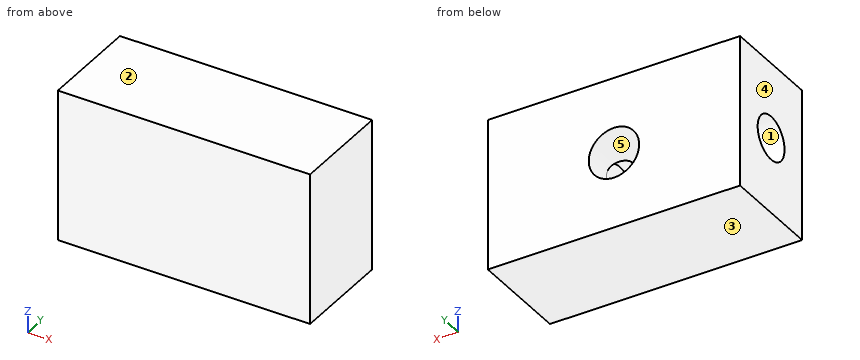
```python
from build123d import *

# Parameters (mm, degrees)
F0_W     = 127
F0_H     = 76.2
F1_DEPTH = 50.8
F2_R     = 12.7
F3_DEPTH = 38.1
F4_R     = 10.982907
F5_DEPTH = 76.2


with BuildPart() as f1:
    # F0 (on Front) → F1 (new body)
    with BuildSketch(Plane.XZ):
        with Locations((3.876453, -23.385659)):
            Rectangle(F0_W, F0_H)
    extrude(amount=F1_DEPTH)

    # F2 (on face) → F3 (cut)
    with BuildSketch(Plane(origin=(0, 0, 0), x_dir=(-1, 0, 0), z_dir=(0, 1, 0))):
        with Locations((-3.876453, -23.385659)):
            Circle(F2_R)
    extrude(amount=-F3_DEPTH, mode=Mode.SUBTRACT)

    # F4 (on face) → F5 (cut)
    with BuildSketch(Plane(origin=(-59.623547, 0, 0), x_dir=(0, -1, 0), z_dir=(-1, 0, 0))):
        with Locations((25.4, -23.385659)):
            Circle(F4_R)
    extrude(amount=-F5_DEPTH, mode=Mode.SUBTRACT)


solid = f1.part
```
Geometry check sheet. Reference: the model listing, model coordinates, mm. Face numbers are marked on the shaded views. A direction names the side the tool comes from. Coordinates: 2 decimals unless noted, no trailing zeros. Write each loop counter-clockwise with the first axis right and the second up, starting at its lowest first coordinate (ties: lowest second). Pieces come first, ordered by that corner, then holes. Notation, with made-up numbers: (77.5, 77) -> (108.5, 77) arc R11 ccw to (108.5, 97) -> close; hole circle Ø7 at (25, 12). An arc over 180 degrees is marked (long way). Use CSV: the item, a comma, the result in double quotes. Start each with the question number.
Item 1: Cross-section at B-B, the plane y = -10.5. Record the cut outline in (x, z), plus the area to 3 significant figures.
Item 2: Thickness scan on line 1 (X direction, y = -12, z = -23); line 2 (Z direction, x = -25.5, y = -25.4); line 3 (X direction, y = -9, z = -25.5). Record the ranges inside material, lowest first.
Item 3: Mould release check, pull along Z, two halves, no side actions. Record for the marked faces 3, 4 and 5: released by +Z, released by -Z, zero draft, split by the parting line, or undercut.
Item 4: Cross-section at A-A, the plane z = -19. Record the cut outline in (x, y).
Item 5: Depth check by flat-ended pin: pin 1 Ø6.5 at (y, z) = (-28.5, -18) entering from -X; pin 2 Ø7.5 at (x, z) = (2.5, -29) entering from +Y. Enter the tip coordinate at first touch or a pass-through.
Item 6: Cross-section at C-C, the plane x = -27. Record the cut outline in (y, z), plus the area to 3 significant figures.
Item 7: Cross-section at D-D, the plane y = -25.4. Record the cut outline in (x, z), plus the area to 3 significant figures.
Item 8: Set-up check for the marked faces 1 and 2: record each of +Z, -Z, +X, -X, +Y, -Y from which the full face is reachable in a straight line by a thin tool's end or side.
Answers:
1,outline,"(-59.62, -61.49) -> (67.38, -61.49) -> (67.38, 14.71) -> (-59.62, 14.71) -> close; hole circle Ø25.4 at (3.88, -23.39)"
1,area,"9,170 mm^2"
2,line 1,"-59.62 to -8.82, 16.57 to 67.38"
2,line 2,"-61.49 to -34.37, -12.4 to 14.71"
2,line 3,"-59.62 to -8.65, 16.4 to 67.38"
3,face 3,"released by -Z"
3,face 4,"zero draft"
3,face 5,"undercut"
4,outline,"(-59.62, -50.8) -> (67.38, -50.8) -> (67.38, 0) -> (15.8, 0) -> (15.8, -15.33) -> (16.58, -15.33) -> (16.58, -35.47) -> (15.8, -35.47) -> (15.8, -38.1) -> (-8.04, -38.1) -> (-8.04, -35.47) -> (-59.62, -35.47) -> close; (-59.62, -15.33) -> (-8.04, -15.33) -> (-8.04, 0) -> (-59.62, 0) -> close"
5,pin 1,"x = 16.58"
5,pin 2,"y = -38.1"
6,outline,"(-50.8, -61.49) -> (0, -61.49) -> (0, 14.71) -> (-50.8, 14.71) -> close; hole circle Ø21.97 at (-25.4, -23.39)"
6,area,"3,490 mm^2"
7,outline,"(-59.62, -61.49) -> (67.38, -61.49) -> (67.38, 14.71) -> (-59.62, 14.71) -> (-59.62, -12.4) -> (-2.5, -12.4) arc R12.7 cw to (10.25, -12.4) -> (16.58, -12.4) -> (16.58, -34.37) -> (10.25, -34.37) arc R12.7 cw to (-2.5, -34.37) -> (-59.62, -34.37) -> close"
7,area,"7,970 mm^2"
8,face 1,"-X"
8,face 2,"+Z, +X, -X, +Y, -Y"
